Autodesk Inventor part; units mm, degrees
ref_plane "YZ Plane" through (0, 0, 0) normal (1, 0, 0) x (0, 1, 0)
ref_plane "XZ Plane" through (0, 0, 0) normal (0, 1, 0) x (-1, 0, 0)
ref_plane "XY Plane" through (0, 0, 0) normal (0, 0, 1) x (1, 0, 0)
sketch "Sketch1" plane through (0, 0, 0) normal (0, 1, 0) x (-1, 0, 0)
  circle A0 centre (0, 0) radius 3.5
  dimension "d0" = 7
extrude "Extrusion1" add sketch "Sketch1" along normal blind 75
sketch "Sketch2" plane through (0, 75, 0) normal (0, 1, 0) x (1, 0, 0)
  circle A0 centre (0, 0) radius 3.5
hole "Hole1" at (0, 75, 0) direction (0, -1, 0) diameter 3.242 depth 10
sketch "Sketch3" plane through (0, 0, 0) normal (0, -1, 0) x (1, 0, 0)
  circle A0 centre (0, 0) radius 3.5
hole "Hole2" at (0, 0, 0) direction (0, 1, 0) diameter 3.242 depth 10
properties part number "214.3"
Build history of the part. All positions in model axes, mm. A direction names the side the tool comes from. Coordinates: 2 decimals unless noted, no trailing zeros. Order: outer loops, then holes, each group sorted by start corner. A loop starts at its lowest first (then second) coordinate and runs counter-clockwise, first axis right, second up. Notation, with made-up numbers: (1.25, 6.25) - (10.25, 6.25) arc R33 ccw to (10.25, 36.25) - close; hole circle Ø7 at (51.25, 59). An arc over 180 degrees is marked (long way). Write item = value, one per line. Start each with the question number.
1) Saw through at C-C on y = 7. Write the cut outline in (x, z).
2) 3-axis set-ups, long thin cutter, end or side, ignore diameter. For faces 1 (the face through (0, 10, 0)), 2 (the face through (0, 65, 0)), 3 (the face through (-1, 75, -2)): which of +Z, -Z, +X, -X, +Y, -Y reach the whole face in a straight line?
3) Wall check: line 1 along Z through (x, y) = (0, 5.5); line 2 along Z through (x, y) = (0.25, 29); line 3 along Y through (x, z) = (1, 0.25). Give the ranges that are in metal, low to high. Write a range as from..to.
4) Two-plate mould, pull along Z, no slides. Class faces 4 (the face through (1.438, 5.07, -0.748)), 5 (the face through (-1, 0, -2)), 6 (the face through (-3.233, 36.975, 1.341)): pulls with the +Z half, pulls with the -Z half, needs draft (parallel to the pull), parting line crosses it, or undercut.
5) Saw through at A-A on x = 0. Write the cut outline in (y, z).
6) Flat gauge pins, fed straight in: pin 1 Ø1 at (y, z) = (56, -2.5) entering from +X; pin 2 Ø1 at (x, y) = (-0.5, 36) entering from +Z; pin 3 Ø2.5 at (x, z) = (0, 0) entering from -Y; pin 4 Ø1.6 at (x, z) = (0, 0.5) entering from +Y. Where does each tip first touch, or does it go through?
7) Saw through at D-D on y = 37. Write the cut outline in (x, z).
8) Saw through at B-B on z = 0. Write the cut outline in (x, y).
From the geometry:
q1.outline = circle Ø7 at (0, 0); hole circle Ø3.24 at (0, 0)
q2.face_1 = -Y
q2.face_2 = +Y
q2.face_3 = +Z, -Z, +X, -X, +Y
q3.line_1 = -3.5..-1.62, 1.62..3.5
q3.line_2 = -3.49..3.49
q3.line_3 = 10..65
q4.face_4 = undercut
q4.face_5 = needs draft
q4.face_6 = parting line crosses it
q5.outline = (0, -3.5) - (75, -3.5) - (75, -1.62) - (65, -1.62) - (65, 1.62) - (75, 1.62) - (75, 3.5) - (0, 3.5) - (0, 1.62) - (10, 1.62) - (10, -1.62) - (0, -1.62) - close
q6.pin_1 = 2.87
q6.pin_2 = 3.5
q6.pin_3 = 10
q6.pin_4 = 65
q7.outline = circle Ø7 at (0, 0)
q8.outline = (-3.5, 0) - (-1.62, 0) - (-1.62, 10) - (1.62, 10) - (1.62, 0) - (3.5, 0) - (3.5, 75) - (1.62, 75) - (1.62, 65) - (-1.62, 65) - (-1.62, 75) - (-3.5, 75) - close
